Work out the finished part from the listing and answer in its coordinate system (mm). A direction names the side the tool comes from. Coordinates: 2 decimals unless noted, no trailing zeros. Order: outer loops, then holes, each group sorted by start corner. A loop starts at its lowest first (then second) coordinate and runs counter-clockwise, first axis right, second up. Notation, with made-up numbers: (70, 22.25) -> (78, 22.25) arc R17 ccw to (78, 30.25) -> close; hole circle Ø11 at (-2.5, -8.75). An arc over 180 degrees is marked (long way). Answer as CSV lines item,"result". Start each with the question number.
Item 1: Which of the six approach directions +Z, -Z, +X, -X, +Y, -Y give full straight-line access (tool end or side, diameter ignored) to faces 1 (the face through (3, 12.7, -1)), 2 (the face through (36.44, -3.13, -1.95))?
Item 2: Section C-C (y = -3.75) is taken. Write down the section's boundary in (x, z), then the cut area to 3 significant figures.
Item 3: Section A-A (x = 31.75) is taken. Write down the section's boundary in (y, z), then the cut area to 3 significant figures.
Item 4: Section B-B (z = 0) is taken. Write down the section's boundary in (x, y), then the cut area to 3 significant figures.
Item 5: This flat-tipped pin is pushed along its axis until it touches: pin 1 Ø6 at (x, z) = (32.5, 12.5) entering from -Y. Where does it stop, or does it pass through?
Item 6: Straight lines are drawn through the part: L1, parallel to Y at x = 6, z = 11; L2, parallel to X at y = -3.5, z = 3.5. For each, find the intervals that lie inside material, in ascending order.
Item 7: Section D-D (z = -25) is taken. Write down the section's boundary in (x, y), then the cut area to 3 significant figures.
Item 8: For a pull along X with two mould halves and no side action, classify faces 3 (the face through (-26.905, -3.131, 1.526)), 4 (the face through (61.33, 6, -2)), 5 (the face through (32, -6.35, 0)) as pulls with the +X half, pulls with the -X half, needs draft (parallel to the pull), parting line crosses it, or undercut.
```python
from build123d import *

# Parameters (mm, degrees)
F0_W     = 115.562398
F0_H     = 74.107583
F1_DEPTH = 12.7
F2_R     = 5.08
F3_DEPTH = 6.35


with BuildPart() as f1:
    # F0 (on Front) → F1 (new body)
    with BuildSketch(Plane.XZ):
        with Locations((3.549216, -1.419687)):
            Rectangle(F0_W, F0_H)
    extrude(amount=-F1_DEPTH)

    # F2 (on Front) → F3 (join)
    with BuildSketch(Plane.XZ):
        with Locations((-31.75, 0)):
            Circle(F2_R)
        with Locations((31.75, 0)):
            Circle(F2_R)
    extrude(amount=F3_DEPTH)


solid = f1.part
```
Checked values:
1,face 1,"+Z, -Z, +X, -X, +Y"
1,face 2,"-Y"
2,outline,"circle Ø10.16 at (-31.75, 0); circle Ø10.16 at (31.75, 0)"
2,area,"162 mm^2"
3,outline,"(-6.35, -5.08) -> (0, -5.08) -> (0, -38.47) -> (12.7, -38.47) -> (12.7, 35.63) -> (0, 35.63) -> (0, 5.08) -> (-6.35, 5.08) -> close"
3,area,"1,010 mm^2"
4,outline,"(-54.23, 0) -> (-36.83, 0) -> (-36.83, -6.35) -> (-26.67, -6.35) -> (-26.67, 0) -> (26.67, 0) -> (26.67, -6.35) -> (36.83, -6.35) -> (36.83, 0) -> (61.33, 0) -> (61.33, 12.7) -> (-54.23, 12.7) -> close"
4,area,"1,600 mm^2"
5,pin 1,"stops at y = 0"
6,L1,"y = 0 to 12.7"
6,L2,"x = -35.43 to -28.07, 28.07 to 35.43"
7,outline,"(-54.23, 0) -> (61.33, 0) -> (61.33, 12.7) -> (-54.23, 12.7) -> close"
7,area,"1,470 mm^2"
8,face 3,"undercut"
8,face 4,"pulls with the +X half"
8,face 5,"needs draft"
